```python
from build123d import *

# Parameters (mm, degrees)
BASPROSKE_W     = 12
BASPROSKE_H     = 33.75
TOOTHCUT_DEPTH  = 50.21508915
TEETHCUTS_COUNT = 25
TEETHCUTS_ANGLE = 345.6
BORSKE_R        = 7.5
BORE_DEPTH      = 50.000508
SCALE2_SCALE    = 0.8


with BuildPart() as part:
    # BasProSke → Base-Revolve (revolve)
    with BuildSketch(Plane(origin=(0, 0, 0), x_dir=(1, 0, 0), z_dir=(0, 1, 0)), mode=Mode.PRIVATE) as base_revolve_sk:
        with Locations((6, 16.875)):
            Rectangle(BASPROSKE_W, BASPROSKE_H)
    revolve(base_revolve_sk.sketch.rotate(Axis((-10, 0, 0), (1, 0, 0)), 180), axis=Axis((-10, 0, 0), (1, 0, 0)))

    # TooCutSke → ToothCut (cut, through all)
    with BuildSketch(Plane(origin=(0, 0, 0), x_dir=(0, 0, -1), z_dir=(1, 0, 0))):
        with BuildLine():
            ThreePointArc((1.187856988, 28.098903391), (0, 28.124), (-1.187856988, 28.098903391))
            ThreePointArc((-1.187856988, 28.098903391), (-2.083835169, 31.109603364), (-3.702102288, 33.801870579))
            ThreePointArc((-3.702102288, 33.801870579), (0, 34.004), (3.702102288, 33.801870579))
            ThreePointArc((3.702102288, 33.801870579), (2.083835169, 31.109603364), (1.187856988, 28.098903391))
        make_face()
    toothcut = extrude(amount=TOOTHCUT_DEPTH, mode=Mode.SUBTRACT)

    # TeethCuts: ToothCut ×25 about axis
    teethcuts_axis = Axis((-10, 0, 0), (1, 0, 0))
    for i in range(1, TEETHCUTS_COUNT):
        add(toothcut.rotate(teethcuts_axis, i * TEETHCUTS_ANGLE / (TEETHCUTS_COUNT - 1)), mode=Mode.SUBTRACT)

    # BorSke → Bore (cut, symmetric)
    with BuildSketch(Plane(origin=(0, 0, 0), x_dir=(0, 0, -1), z_dir=(1, 0, 0))):
        with Locations(Location((0, 0, 0), (0, 0, 180))):
            Circle(BORSKE_R)
    extrude(amount=BORE_DEPTH, both=True, mode=Mode.SUBTRACT)


with BuildPart() as part_1:
    # Scale2: scaled about (6, 0, 0)
    add(part.part.scale(SCALE2_SCALE).moved(Location((1.2, 0, 0))))


solid = part_1.part
```
Here's how the part is built. I have some questions about the finished solid (model axes, mm). A direction names the side the tool comes from. Give positions to 0.01 mm unless a question says otherwise; leave off trailing zeros. Order: outer loops, then holes, each group sorted by start corner. A loop starts at its lowest first (then second) coordinate and runs counter-clockwise, first axis right, second up. Notation, with made-up numbers: (2.25, 11) - (19.25, 11) arc R17 cw to (19.25, 41) - close; hole circle Ø1 at (42, 3). An arc over 180 degrees is marked (long way). Answer as a JSON object with one key per item and string values. Group by question number.
Item 1: Please list where these lines run through material, in increasing order: probe 1 along Y at (x, z) = (5, 0); probe 2 along Z at (x, y) = (2.25, 23.5); probe 3 along Z at (x, y) = (4.5, 21).
Item 2: Which directions (+Z, -Z, +X, -X, +Y, -Y) give clear straight access to the entire face, cutting with the end or side of a thin tool? Please do faces 4 (the cylindrical face through (5.933, 11.915, -21.822)), 5 (the cylindrical face through (5.93, 23.62, -7.75)), 6 (the cylindrical face through (5.933, -22.466, 10.651)).
Item 3: If we mould it in two halves opening along Z, with no side actions, what happens to faces 1 (the cylindrical face through (5.933, -20.965, 13.247)), 2 (the flat face through (10.8, -6.4, 0.4)), 3 (the cylindrical face through (5.933, -17.013, 18.044))? For each: pulls with the +Z half, pulls with the -Z half, needs draft (parallel to the pull), parting line crosses it, or undercut.
Item 4: For P1, Ø1.5, axis at x = 4, y = 9.5, coming from the -Z side (3 decimals); P2, Ø7, axis at y = 0, z = 0, coming from the +X side; P3, Ø3, axis at x = 8.5, z = -1.5, coming from the -Y side; P4, Ø5, axis at x = 9, y = 9, coming from the +Z side, each with a flat end and sliding along its axis, tell me the tip position at first contact or that it passes through.
Item 5: If we section it at A-A on y = 10: Please give me the cut outline in (x, z), and give its area (3 significant figures).
Result set:
{
 "1": {"probe 1": "-27 to -6, 6 to 22.5", "probe 2": "-10.57 to -7.66, -4.69 to -1.17, 1.17 to 4.69, 7.66 to 10.57", "probe 3": "-16.26 to -13.44, -10.25 to 10.25, 13.44 to 16.26"},
 "2": {"face 4": "+X, -X", "face 5": "+X, -X, +Y", "face 6": "+X, -X, -Y"},
 "3": {"face 1": "undercut", "face 2": "needs draft", "face 3": "pulls with the +Z half"},
 "4": {"P1": "z = -24.105", "P2": "through", "P3": "y = -27", "P4": "z = 24.67"},
 "5": {"outline": "(1.2, -23.88) - (10.8, -23.88) - (10.8, 23.88) - (1.2, 23.88) - close", "area": "459 mm²"}
}
